from build123d import *


with BuildPart() as f1:
    # F0 (on Front) → F1 (revolve)
    with BuildSketch(Plane.XZ):
        with BuildLine():
            Line((151.253424, 11.254308), (29.166639, 13.973743))
            Line((29.166639, 13.973743), (29.166639, 0))
            Line((29.166639, 0), (125.650197, 0))
            ThreePointArc((125.650197, 0), (136.271784, -2.236273), (145.090006, -8.565411))
            ThreePointArc((145.090006, -8.565411), (155.771268, -15.34929), (168.415868, -15.82308))
            Line((168.415868, -15.82308), (332.77935, 22.097347))
            ThreePointArc((332.77935, 22.097347), (336.331788, 27.680104), (330.806913, 31.321911))
            Line((330.806913, 31.321911), (184.299229, 3.137134))
            ThreePointArc((184.299229, 3.137134), (166.888073, 3.579557), (151.253424, 11.254308))
        make_face()
    revolve(axis=Axis((29.166639, 0, 0.612669), (0, 0, -1)))


solid = f1.part
Input: part model. Units: mm. Frame: model coordinates. A direction names the side the tool comes from. Round coordinates to 2 decimals unless told otherwise and drop trailing zeros. Use a Markdown table: item, result.
1. Access query for faces 1 (the face through (31, -1, 0)), 2 (the face through (31.9, 5.26, 13.84)). Directions: +Z, -Z, +X, -X, +Y, -Y. A direction counts if a zero-diameter tool reaches every point of the face in a straight line with its end or side. Return the directions, or none.
Evaluation:
| item | result |
|---|---|
| face 1 | -Z |
| face 2 | +Z |
2. Mould query, pull axis X, two halves, no side actions, for faces 3 (the face through (-3.25, 145.98, -13.45)), 4 (the face through (183.9, -48.7, 4.5)). Classes: +X half, -X half, draft (parallel to the pull), parting line (faces both ways), or undercut.
Evaluation:
| item | result |
|---|---|
| face 3 | parting line |
| face 4 | undercut |
3. Material intervals for probe 1 along Z at (x, y) = (34.5, -228.5); probe 2 along Z at (x, y) = (188, -169), sorted ascending.
Evaluation:
| item | result |
|---|---|
| probe 1 | 4.78 to 17.26 |
| probe 2 | 5.56 to 17.91 |
4. First-contact query: pin 1 (10 mm diameter, centred on x = -95, z = 25.5, fed in from +Y); pin 2 (1.5 mm diameter, centred on x = 35.5, z = 25.5, fed in from +Y); pin 3 (6 mm diameter, centred on y = 107, z = 21, fed in from +X). Flat tips, straight axial feed; report the tip coordinate or a pass-through.
Evaluation:
| item | result |
|---|---|
| pin 1 | y = 283.18 |
| pin 2 | y = 307.18 |
| pin 3 | x = 316.55 |
